Can you work these out from the model? Positions are in its coordinate system, mm. A direction names the side the tool comes from. Give positions to 0.01 mm unless a question says otherwise; leave off trailing zeros. Order: outer loops, then holes, each group sorted by start corner. A loop starts at its lowest first (then second) coordinate and runs counter-clockwise, first axis right, second up. Notation, with made-up numbers: (36.25, -22.5) -> (53.25, -22.5) arc R26 cw to (53.25, 16.5) -> close; hole circle Ø6 at (84.5, -13). An arc over 180 degrees is marked (long way). Answer as a JSON object with one key per item and string values.
```python
from build123d import *

# Parameters (mm, degrees)
F1_DEPTH  = 20
F3_DEPTH  = 50
F5_DEPTH  = 50
F7_DEPTH  = 50
F9_DEPTH  = 50
F11_DEPTH = 50
F13_DEPTH = 50
F15_DEPTH = 25
F17_DEPTH = 25
F19_DEPTH = 25
F21_DEPTH = 25
F23_DEPTH = 25
F25_DEPTH = 25
F27_DEPTH = 5
F28_R     = 4.99999
F29_R     = 1.5
F30_DEPTH = 16.1


# Not quite as in the source:
# - a fillet or chamfer is up to 0.001 mm smaller than in the source, because OpenCascade refuses the exact size


with BuildPart() as f1:
    # F0 (on Top) → F1 (new body)
    with BuildSketch(Plane.XY):
        Polygon((-7.2168783649, 12.5), (-14.4337567297, 0), (-7.2168783649, -12.5), (7.2168783649, -12.5), (14.4337567297, 0), (7.2168783649, 12.5), align=None)
    extrude(amount=F1_DEPTH)

    # F2 (on face) → F3 (join)
    with BuildSketch(Plane.XZ.offset(12.5)):
        with BuildLine():
            Line((0, 10), (7.2168783649, 20))
            add(Edge.make_bspline(
                [(7.2168783649, 20), (3.8943965132, 17.3283502948), (0.5892440485, 14.6441941819), (-1.8163820731, 11.3108608486)],
                knots=[0, 0, 0, 0, 0.5, 0.5, 0.5, 0.5], degree=3))
            Line((-1.8163820731, 11.3108608486), (0, 10))
        make_face()
        with BuildLine():
            Line((-7.2168783649, 0), (0, 10))
            Line((0, 10), (-1.8163820731, 11.3108608486))
            add(Edge.make_bspline(
                [(-1.8163820731, 11.3108608486), (-4.2220081948, 7.9775275153), (-5.7281079733, 3.9950169615), (-7.2168783649, 0)],
                knots=[0.5, 0.5, 0.5, 0.5, 1, 1, 1, 1], degree=3))
        make_face()
    extrude(amount=F3_DEPTH)

    # F4 (on face) → F5 (join)
    with BuildSketch(Plane(origin=(10.8253175473, -6.25, 0), x_dir=(0.5, 0.8660254038, 0), z_dir=(0.8660254038, -0.5, 0))):
        with BuildLine():
            Line((-7.2168783649, 0), (7.2168783649, 20))
            add(Edge.make_bspline(
                [(7.2168783649, 20), (3.8943965132, 17.3283502948), (-2.7159084163, 11.960038069), (-5.7281079733, 3.9950169615), (-7.2168783649, 0)],
                knots=[0, 0, 0, 0, 0.5, 1, 1, 1, 1], degree=3))
        make_face()
    extrude(amount=F5_DEPTH)

    # F6 (on face) → F7 (join)
    with BuildSketch(Plane(origin=(10.8253175473, 6.25, 0), x_dir=(-0.5, 0.8660254038, 0), z_dir=(0.8660254038, 0.5, 0))):
        with BuildLine():
            Line((-7.2168783649, 0), (7.2168783649, 20))
            add(Edge.make_bspline(
                [(7.2168783649, 20), (3.8943965132, 17.3283502948), (-2.7159084163, 11.960038069), (-5.7281079733, 3.9950169615), (-7.2168783649, 0)],
                knots=[0, 0, 0, 0, 0.5, 1, 1, 1, 1], degree=3))
        make_face()
    extrude(amount=F7_DEPTH)

    # F8 (on face) → F9 (join)
    with BuildSketch(Plane(origin=(0, 12.5, 0), x_dir=(-1, 0, 0), z_dir=(0, 1, 0))):
        with BuildLine():
            Line((-7.183146663, 0), (7.2506100667, 20))
            add(Edge.make_bspline(
                [(7.2506100667, 20), (3.9281282151, 17.3283502948), (-2.6821767144, 11.960038069), (-5.6943762714, 3.9950169615), (-7.183146663, 0)],
                knots=[0, 0, 0, 0, 0.5, 1, 1, 1, 1], degree=3))
        make_face()
    extrude(amount=F9_DEPTH)

    # F10 (on face) → F11 (join)
    with BuildSketch(Plane(origin=(-10.8253175473, 6.25, 0), x_dir=(-0.5, -0.8660254038, 0), z_dir=(-0.8660254038, 0.5, 0))):
        with BuildLine():
            Line((-7.2168783649, 0), (7.2168783649, 20))
            add(Edge.make_bspline(
                [(7.2168783649, 20), (3.8943965132, 17.3283502948), (-2.7159084163, 11.960038069), (-5.7281079733, 3.9950169615), (-7.2168783649, 0)],
                knots=[0, 0, 0, 0, 0.5, 1, 1, 1, 1], degree=3))
        make_face()
    extrude(amount=F11_DEPTH)

    # F12 (on face) → F13 (join)
    with BuildSketch(Plane(origin=(-10.8253175473, -6.25, 0), x_dir=(0.5, -0.8660254038, 0), z_dir=(-0.8660254038, -0.5, 0))):
        with BuildLine():
            Line((-7.2168782353, 0), (7.2168784944, 20))
            add(Edge.make_bspline(
                [(7.2168784944, 20), (3.8943966428, 17.3283502948), (-2.7159082867, 11.960038069), (-5.7281078437, 3.9950169615), (-7.2168782353, 0)],
                knots=[0, 0, 0, 0, 0.5, 1, 1, 1, 1], degree=3))
        make_face()
    extrude(amount=F13_DEPTH)

    # F14 (on face) → F15 (cut)
    with BuildSketch(Plane(origin=(-2.3726722966, 4.1095889673, 3.4246574728), x_dir=(0.914120582, 0.3114695001, 0.2595579168), z_dir=(0.405442427, -0.7022468832, -0.585205736))):
        with BuildLine():
            Line((-52.6686272502, 39.3713406512), (-56.6160705917, 27.6879752855))
            Line((-56.6160705917, 27.6879752855), (-51.879138611, 26.0875142863))
            add(Edge.make_bspline(
                [(-51.879138611, 26.0875142863), (-42.9404048496, 29.8743142581), (-24.1198561583, 26.6205224229), (-5.299307467, 23.3667305878)],
                knots=[0.3481274936, 0.3481274936, 0.3481274936, 0.3481274936, 1, 1, 1, 1], degree=3))
            Line((-5.2993074428, 23.3667306596), (-52.6686272502, 39.3713406512))
        make_face()
        with BuildLine():
            Line((-51.879138611, 26.0875142863), (-56.6160705917, 27.6879752855))
            Line((-56.6160705917, 27.6879752855), (-60.5635138847, 16.0046100634))
            add(Edge.make_bspline(
                [(-60.563513909, 16.0046099916), (-58.608157235, 20.034906453), (-56.6528005609, 24.0652029143), (-51.879138611, 26.0875142863)],
                knots=[0, 0, 0, 0, 0.3481274936, 0.3481274936, 0.3481274936, 0.3481274936], degree=3))
        make_face()
    extrude(amount=-F15_DEPTH, mode=Mode.SUBTRACT)

    # F16 (on face) → F17 (cut)
    with BuildSketch(Plane(origin=(-4.7453446783, 0, 3.4246575342), x_dir=(0, 1, 0), z_dir=(0.8108848541, 0, -0.585205736))):
        with BuildLine():
            Line((-62.5, 20.4410556966), (-62.5, 8.1088485408))
            Line((-62.5, 8.1088485408), (-57.5, 8.1088485408))
            add(Edge.make_bspline(
                [(-57.5, 8.1088485408), (-50.2436903689, 14.5576302724), (-31.3718451845, 17.4993429845), (-12.5, 20.4410556966)],
                knots=[0.3481274936, 0.3481274936, 0.3481274936, 0.3481274936, 1, 1, 1, 1], degree=3))
            Line((-12.5, 20.4410556966), (-62.5, 20.4410556966))
        make_face()
        with BuildLine():
            Line((-57.5, 8.1088485408), (-62.5, 8.1088485408))
            Line((-62.5, 8.1088485408), (-62.5, -4.223358615))
            add(Edge.make_bspline(
                [(-62.5, -4.223358615), (-61.9375881477, 0.2207838442), (-61.3751762953, 4.6649263034), (-57.5, 8.1088485408)],
                knots=[0, 0, 0, 0, 0.3481274936, 0.3481274936, 0.3481274936, 0.3481274936], degree=3))
        make_face()
    extrude(amount=-F17_DEPTH, mode=Mode.SUBTRACT)

    # F18 (on face) → F19 (cut)
    with BuildSketch(Plane(origin=(-2.3726723391, -4.1095890411, 3.4246575342), x_dir=(-0.914120582, 0.3114695001, -0.2595579168), z_dir=(0.405442427, 0.7022468832, -0.585205736))):
        with BuildLine():
            Line((-65.7546722441, -0.6401843997), (-61.8072289268, -12.3235496935))
            Line((-61.8072289268, -12.3235496935), (-57.070296946, -10.7230886944))
            add(Edge.make_bspline(
                [(-57.070296946, -10.7230886944), (-52.259972646, -2.2909124977), (-35.3226625414, 6.5367565471), (-18.3853524367, 15.3644255919)],
                knots=[0.3481274936, 0.3481274936, 0.3481274936, 0.3481274936, 1, 1, 1, 1], degree=3))
            Line((-18.3853524367, 15.3644255919), (-65.7546722441, -0.6401843997))
        make_face()
        with BuildLine():
            Line((-57.070296946, -10.7230886944), (-61.8072289268, -12.3235496935))
            Line((-61.8072289268, -12.3235496935), (-57.8597856095, -24.0069149874))
            add(Edge.make_bspline(
                [(-57.8597856095, -24.0069149874), (-58.7494996077, -19.616571232), (-59.6392136059, -15.2262274766), (-57.070296946, -10.7230886944)],
                knots=[0, 0, 0, 0, 0.3481274936, 0.3481274936, 0.3481274936, 0.3481274936], degree=3))
        make_face()
    extrude(amount=-F19_DEPTH, mode=Mode.SUBTRACT)

    # F20 (on face) → F21 (cut)
    with BuildSketch(Plane(origin=(2.3726723391, -4.1095890411, 3.4246575342), x_dir=(-0.914120582, -0.3114695001, 0.2595579168), z_dir=(-0.405442427, 0.7022468832, -0.585205736))):
        with BuildLine():
            Line((-52.6686272744, 39.3713405794), (-56.6160705917, 27.6879752855))
            Line((-56.6160705917, 27.6879752855), (-51.879138611, 26.0875142863))
            add(Edge.make_bspline(
                [(-51.879138611, 26.0875142863), (-42.9404048496, 29.8743142581), (-24.1198561583, 26.6205224229), (-5.299307467, 23.3667305878)],
                knots=[0.3481274936, 0.3481274936, 0.3481274936, 0.3481274936, 1, 1, 1, 1], degree=3))
            Line((-5.299307467, 23.3667305878), (-52.6686272744, 39.3713405794))
        make_face()
        with BuildLine():
            Line((-51.879138611, 26.0875142863), (-56.6160705917, 27.6879752855))
            Line((-56.6160705917, 27.6879752855), (-60.563513909, 16.0046099916))
            add(Edge.make_bspline(
                [(-60.563513909, 16.0046099916), (-58.608157235, 20.034906453), (-56.6528005609, 24.0652029143), (-51.879138611, 26.0875142863)],
                knots=[0, 0, 0, 0, 0.3481274936, 0.3481274936, 0.3481274936, 0.3481274936], degree=3))
        make_face()
    extrude(amount=-F21_DEPTH, mode=Mode.SUBTRACT)

    # F22 (on face) → F23 (cut)
    with BuildSketch(Plane(origin=(4.7231649291, 0, 3.4086506791), x_dir=(0, -1, 0), z_dir=(-0.8108848541, 0, -0.585205736))):
        with BuildLine():
            Line((-62.5, 20.460795682), (-62.5, 8.1285885262))
            Line((-62.5, 8.1285885262), (-57.5, 8.1285885262))
            add(Edge.make_bspline(
                [(-57.5, 8.1285885262), (-50.2436903689, 14.5773702578), (-31.3718451845, 17.5190829699), (-12.5, 20.460795682)],
                knots=[0.3481274936, 0.3481274936, 0.3481274936, 0.3481274936, 1, 1, 1, 1], degree=3))
            Line((-12.5, 20.460795682), (-62.5, 20.460795682))
        make_face()
        with BuildLine():
            Line((-57.5, 8.1285885262), (-62.5, 8.1285885262))
            Line((-62.5, 8.1285885262), (-62.5, -4.2036186296))
            add(Edge.make_bspline(
                [(-62.5, -4.2036186296), (-61.9375881477, 0.2405238296), (-61.3751762953, 4.6846662888), (-57.5, 8.1285885262)],
                knots=[0, 0, 0, 0, 0.3481274936, 0.3481274936, 0.3481274936, 0.3481274936], degree=3))
        make_face()
    extrude(amount=-F23_DEPTH, mode=Mode.SUBTRACT)

    # F24 (on face) → F25 (cut)
    with BuildSketch(Plane(origin=(2.3726723391, 4.1095890411, 3.4246575342), x_dir=(0.914120582, -0.3114695001, -0.2595579168), z_dir=(-0.405442427, -0.7022468832, -0.585205736))):
        with BuildLine():
            Line((-65.7546722441, -0.6401843997), (-61.8072289268, -12.3235496935))
            Line((-61.8072289268, -12.3235496935), (-57.070296946, -10.7230886944))
            add(Edge.make_bspline(
                [(-57.070296946, -10.7230886944), (-52.259972646, -2.2909124977), (-35.3226625414, 6.5367565471), (-18.3853524367, 15.3644255919)],
                knots=[0.3481274936, 0.3481274936, 0.3481274936, 0.3481274936, 1, 1, 1, 1], degree=3))
            Line((-18.3853524367, 15.3644255919), (-65.7546722441, -0.6401843997))
        make_face()
        with BuildLine():
            Line((-57.070296946, -10.7230886944), (-61.8072289268, -12.3235496935))
            Line((-61.8072289268, -12.3235496935), (-57.8597856095, -24.0069149874))
            add(Edge.make_bspline(
                [(-57.8597856095, -24.0069149874), (-58.7494996077, -19.616571232), (-59.6392136059, -15.2262274766), (-57.070296946, -10.7230886944)],
                knots=[0, 0, 0, 0, 0.3481274936, 0.3481274936, 0.3481274936, 0.3481274936], degree=3))
        make_face()
    extrude(amount=-F25_DEPTH, mode=Mode.SUBTRACT)

    # F26 (on face) → F27 (join)
    with BuildSketch(Plane.XY.offset(20)):
        with BuildLine():
            ThreePointArc((10.8253174264, -6.2500002094), (12.0740727973, -3.2352381805), (12.5, 0))
            ThreePointArc((12.5, 0), (12.0740728368, 3.2352380332), (10.825317579, 6.2499999451))
            ThreePointArc((10.825317579, 6.2499999451), (6.2500000275, 10.8253175315), (0, 12.5))
            ThreePointArc((0, 12.5), (-6.2500001608, 10.8253174545), (-10.825317733, 6.2499996783))
            ThreePointArc((-10.825317733, 6.2499996783), (-12.5, -1.905e-07), (-10.8253175425, -6.2500000083))
            ThreePointArc((-10.8253175425, -6.2500000083), (-6.2499999958, -10.8253175497), (0, -12.5))
            ThreePointArc((0, -12.5), (6.2499998953, -10.8253176077), (10.8253174264, -6.2500002094))
        make_face()
    extrude(amount=F27_DEPTH)

    # F28 (radius 5 in the source; OpenCascade refuses exactly that, so slightly less here)
    f28_edges = [f1.edges().sort_by_distance(p)[0] for p in [
        (10.825318, 6.25, 25),
    ]]
    fillet(f28_edges, radius=F28_R)

    # F29 (on face) → F30 (cut)
    with BuildSketch(Plane(origin=(0, 0, 0), x_dir=(1, 0, 0), z_dir=(0, 0, -1))):
        Circle(F29_R)
    extrude(amount=-F30_DEPTH, mode=Mode.SUBTRACT)


solid = f1.part
```
1. Please list where these lines run through material, in increasing order: L1, parallel to X at y = 0, z = 6.5; L2, parallel to Y at x = 0, z = 4; L3, parallel to X at y = -17, z = 10.25.
Worked answers:
{"L1": "-14.43 to -1.5, 1.5 to 14.43", "L2": "-12.5 to -1.5, 1.5 to 12.5", "L3": "-34.52 to -29.08, -2.54 to 0.18, 24.37 to 29.81"}
2. For faces 1 (the face through (-1.5, -0.07, 7.94)), 2 (the face through (3, -12.5, 5)), 3 (the face through (9.27, 8.94, 5.42)), 4 (the face through (-6.2, -11.2, 20)), which set-ups out of +Z, -Z, +X, -X, +Y, -Y let a thin tool reach every point of the face, with its end or its side?
Worked answers:
{"face 1": "-Z", "face 2": "-Z, -Y", "face 3": "-Z, +Y", "face 4": "+Z, -X, -Y"}
3. If we mould it in two halves opening along X, with no side actions, what happens to faces 5 (the face through (-9.27, -8.94, 5.42)), 6 (the face through (26.5, -17.3, 7.6)), 7 (the face through (7, 11, 20)), 8 (the face through (-12.38, 3.56, 5.42))? For each: +X half, -X half, draft (parallel to the pull), parting line (faces both ways), or undercut.
Worked answers:
{"face 5": "undercut", "face 6": "+X half", "face 7": "draft", "face 8": "-X half"}
4. Will these pins go through, and if not, where does the flat tip stop? pin 1 Ø3 at (x, y) = (6.5, 10.5) entering from +Z; pin 2 Ø1.5 at (x, y) = (28.5, -22.5) entering from -Z; pin 3 Ø8 at (y, z) = (25.5, 12.5) entering from +X; pin 4 Ø3 at (x, y) = (45, -36.5) entering from +Z.
Worked answers:
{"pin 1": "z = 23.71", "pin 2": "z = 1.71", "pin 3": "x = 53.63", "pin 4": "through"}
5. If we section it at A-A on z = 22: Please give me the cut outline in (x, y), then the cut area to 3 significant figures.
Worked answers:
{"outline": "circle Ø24.17 at (0, 0)", "area": "459 mm²"}
